Source: CAD feature listing. Evaluate the final solid. Frame: model axes, mm. A direction names the side the tool comes from. Round coordinates to 2 decimals unless told otherwise and drop trailing zeros. Loops run counter-clockwise (first coordinate to the right, second up) from the corner with the lowest first, then second, coordinate; pieces in that order, holes last. Notation, with made-up numbers: M -6,14 L 51,14 A37 cw 51,52 Z; hole C 29,23.5 d5. An arc over 180 degrees is marked long. Answer as a JSON object with one key per item and string values.
from build123d import *


with BuildPart() as part:
    # 草图1 → 旋转3 (revolve)
    with BuildSketch(Plane.XY, mode=Mode.PRIVATE) as revolve_3_sk:
        Polygon((0, 3.5), (0, 0), (10, 0), (10, 7.5), (3, 7.5), (3, 3.5), align=None)
        Polygon((10, 0), (0, 0), (0, -3.5), (3, -3.5), (3, -7.5), (10, -7.5), align=None)
    revolve(revolve_3_sk.sketch.rotate(Axis((0, 3.5, 0), (0, -1, 0)), 180), axis=Axis((0, 3.5, 0), (0, -1, 0)))


solid = part.part
Item 1: Contact query for flat-ended pins moving along their axis: pin 1 Ø3.5 at (x, z) = (0, 0) entering from +Y; pin 2 Ø1 at (y, z) = (5.5, -1) entering from +X; pin 3 Ø2 at (y, z) = (2.5, -5) entering from +X. Output: stop coordinate, or through.
Answer sheet:
{"pin 1": "stops at y = 3.5", "pin 2": "stops at x = 9.99", "pin 3": "stops at x = 9.17"}
Item 2: Section B-B on z = 0. Return the cut outline in (x, y), then the cut area to 3 significant figures.
Answer sheet:
{"outline": "M -10,-7.5 L -3,-7.5 L -3,-3.5 L 3,-3.5 L 3,-7.5 L 10,-7.5 L 10,7.5 L 3,7.5 L 3,3.5 L -3,3.5 L -3,7.5 L -10,7.5 Z", "area": "252 mm²"}
Item 3: Access query for faces 1 (the cylindrical face through (-2.86, 5.47, -0.9)), 2 (the cylindrical face through (-2.86, -5.53, -0.9)), 3 (the flat face through (2.1, -7.5, -2.4)). Directions: +Z, -Z, +X, -X, +Y, -Y. A direction counts if a zero-diameter tool reaches every point of the face in a straight line with its end or side. Return the directions, or none.
Answer sheet:
{"face 1": "+Y", "face 2": "-Y", "face 3": "+Z, -Z, +X, -X, -Y"}
Item 4: Line query: probe 1 along Z at (x, y) = (0, 4.35); probe 2 along X at (y, z) = (6.5, 2.5); probe 3 along X at (y, z) = (-6, -2.75). Output: solid intervals per line, ascending. Write a range as from..to.
Answer sheet:
{"probe 1": "z = -10..-3, 3..10", "probe 2": "x = -9.68..-1.66, 1.66..9.68", "probe 3": "x = -9.61..-1.2, 1.2..9.61"}
Item 5: Section D-D on x = 6. Return the cut outline in (y, z), then the cut area to 3 significant figures.
Answer sheet:
{"outline": "M -7.5,-8 L 7.5,-8 L 7.5,8 L -7.5,8 Z", "area": "240 mm²"}
Item 6: Pull-direction query (X, two-part tool) for faces 4 (the cylindrical face through (10, 0, 0)), 5 (the flat face through (-2.1, 7.5, -2.4)), 6 (the flat face through (0, 3.5, 0)), 7 (the flat face through (0, -3.5, 0)); classes: pulls with the +X half, pulls with the -X half, needs draft (parallel to the pull), parting line crosses it, or undercut.
Answer sheet:
{"face 4": "parting line crosses it", "face 5": "needs draft", "face 6": "undercut", "face 7": "undercut"}
Item 7: Section C-C on y = 3. Return the cut outline in (x, z).
Answer sheet:
{"outline": "C 0,0 d20"}
Item 8: Section A-A on x = 0. Return the cut outline in (y, z), then the cut area to 3 significant figures.
Answer sheet:
{"outline": "M -7.5,-10 L 7.5,-10 L 7.5,-3 L 3.5,-3 L 3.5,3 L 7.5,3 L 7.5,10 L -7.5,10 L -7.5,3 L -3.5,3 L -3.5,-3 L -7.5,-3 Z", "area": "252 mm²"}
